The model under review builds one solid part; all positions refer to its coordinate system, in mm. A direction names the side the tool comes from. Coordinates: 2 decimals unless noted, no trailing zeros. Write each loop counter-clockwise with the first axis right and the second up, starting at its lowest first coordinate (ties: lowest second). Pieces come first, ordered by that corner, then holes. Notation, with made-up numbers: (76.25, 81.25) - (92.25, 81.25) arc R14 ccw to (92.25, 100.25) - close; hole circle Ø1 at (-17.75, 27). An arc over 180 degrees is marked (long way). Put each result on its own line as item: value. Start each with the question number.
Item 1: For pin 1 (4 mm diameter, centred on y = 12, z = 21, fed in from -X); pin 2 (8 mm diameter, centred on x = -29.11, y = 108.35, fed in from +Z); pin 3 (7 mm diameter, centred on x = -2, y = 31, fed in from +Z); pin 4 (10 mm diameter, centred on y = 57, z = 38.5, fed in from -X), all flat-tipped, find the tip position at first contact; note any pin that passes through.
Item 2: Consider section D-D on z = 12. Give the boundary of the cut face in (x, y), then the cut area to 3 significant figures.
Item 3: Mouldability with a two-part tool opening along Y and no side actions: class faces 5 (the face through (-0.2, -5.4, 58)), 6 (the face through (1.365, 57.131, 27.863)), 7 (the face through (25.337, -0.132, 30.461)), 8 (the face through (-5.521, 32.274, 27.579)) as pulls with the +Y half, pulls with the -Y half, needs draft (parallel to the pull), parting line crosses it, or undercut.
Item 4: Machinability: for faces 1 (the face through (-6.24, 13.99, 40.49)), 2 (the face through (-19.001, 80.656, 21.719)), 3 (the face through (-4, 26.69, 36.6)), 4 (the face through (-6.39, 13.17, 35.59)), which of the approach directions +Z, -Z, +X, -X, +Y, -Y give a long, thin tool a straight path to every point of the face, cutting with its end or side? Answer none if there is none.
Item 5: Consider section A-A on y = 0. Give the boundary of the cut face in (x, z).
Item 6: To check wall thickness, follow L1, parallel to Y at x = 0, z = 4; L2, parallel to Y at x = 82, z = 31; L3, parallel to Z at x = 126, y = 0. State the ranges of each line that lie inside material, in increasing order. Write a range as [from, to].
Item 7: Consider section C-C on y = 32. Give the boundary of the cut face in (x, z), then the cut area to 3 significant figures.
Solid Edge part; units mm, degrees
sketch "Sketch1" plane through (0, 0, 0) normal (0, 0, 1) x (1, 0, 0)
  circle A0 centre (0, 0) radius 12.5
extrude "Protrusion1" add sketch "Sketch1" along normal blind 58
sketch "Sketch2" plane through (0, 0, 0) normal (1, 0, 0) x (0, 1, 0)
  circle A0 centre (0, 30.6149) radius 11
extrude "ExtrudedProtrusion_2" add sketch "Sketch2" along normal blind 135
sketch "Sketch3" plane through (0, 0, 58) normal (0, 0, 1) x (1, 0, 0)
  circle A0 centre (0, 0) radius 5
extrude "ExtrudedCutout_1" cut sketch "Sketch3" against normal blind 74.8467
cosmetic_thread "Thread_1" thread depth 22
sketch "Sketch4" plane through (0, 0, 0) normal (0, 0, 1) x (1, 0, 0)
  circle A0 centre (28.334, 0) radius 3
extrude "ExtrudedCutout_2" cut sketch "Sketch4" along normal blind 57.1507
sketch "Sketch5" plane through (0, 0, 19.1008) normal (0, 0, 1) x (1, 0, 0)
  arc A0 (-10.1543, 6) -> (10.1543, 6) centre (0, 0) cw
  line L0 (19.7049, 60.1644) -> (10.1543, 6)
  line L1 (-23.2319, 115.4494) -> (19.7049, 60.1644)
  arc A1 (-33.0541, 116.6842) -> (-23.2319, 115.4494) centre (-28.7604, 111.1557) cw
  line L2 (-36.2132, 114.2307) -> (-33.0541, 116.6842)
  arc A2 (-36.2132, 114.2307) -> (-37.4481, 104.4085) centre (-31.9196, 108.7022) ccw
  line L3 (-1.0629, 57.5595) -> (-37.4481, 104.4085)
  line L4 (-10.1543, 6) -> (-1.0629, 57.5595)
  circle A3 centre (-29.1132, 108.3494) radius 3
  dimension "D1" = 23.2319
  dimension "D2" = 19.7049
  dimension "D3" = 23.2319
extrude "ExtrudedProtrusion_3" add sketch "Sketch5" along normal blind 5.3111
sketch "Sketch6" plane through (-5.5858, 31.9091, 21.7563) normal (-0.9848, 0.1736, 0) x (-0.1736, -0.9848, 0)
  line L0 (24.5955, 2.6555) -> (-26.046, 2.6555)
  line L1 (-26.046, 2.6555) -> (-26.046, 9.6555)
  line L2 (-26.046, 9.6555) -> (24.5955, 28.6555)
  line L3 (24.5955, 28.6555) -> (24.5955, 2.6555)
  line L4 (-6.1187, 8.6555) -> (16.5955, 8.6555)
  arc A0 (16.5955, 8.6555) -> (18.5955, 10.6555) centre (16.5955, 10.6555) ccw
  line L5 (18.5955, 10.6555) -> (18.5955, 17.1095)
  arc A1 (15.893, 18.9821) -> (18.5955, 17.1095) centre (16.5955, 17.1095) cw
  line L6 (15.893, 18.9821) -> (-6.4699, 10.5918)
  arc A2 (-6.4699, 10.5918) -> (-6.1187, 8.6555) centre (-6.1187, 9.6555) ccw
  dimension "D1" = 24.5955
  dimension "D2" = 26.046
extrude "ExtrudedProtrusion_5" add sketch "Sketch6" against normal blind 5
properties material "Steel"
Report:
1. pin 1: x = -9.45
1. pin 2: z = 24.41
1. pin 3: z = 42.6
1. pin 4: through
2. outline: circle Ø25 at (0, 0); hole circle Ø10 at (0, 0)
2. area: 412 mm²
3. face 5: needs draft
3. face 6: pulls with the +Y half
3. face 7: undercut
3. face 8: undercut
4. face 1: none
4. face 2: +Z, -Z, -X
4. face 3: -X
4. face 4: +X
5. outline: (-12.5, 0) - (-5, 0) - (-5, 58) - (-12.5, 58) - close; (5, 0) - (12.5, 0) - (12.5, 19.61) - (25.33, 19.61) - (25.33, 41.61) - (12.5, 41.61) - (12.5, 58) - (5, 58) - close; (31.33, 19.61) - (135, 19.61) - (135, 41.61) - (31.33, 41.61) - close
6. L1: [-12.5, -5], [5, 12.5]
6. L2: [-10.99, 10.99]
6. L3: [19.61, 41.61]
7. outline: (-5.57, 19.1) - (14.74, 19.1) - (14.74, 24.41) - (-0.49, 24.41) - (-0.49, 30.41) - (-5.57, 30.41) - close; (-5.57, 34.74) - (-0.49, 34.41) - (-0.49, 40.82) - (-5.57, 41.15) - close
7. area: 171 mm²
